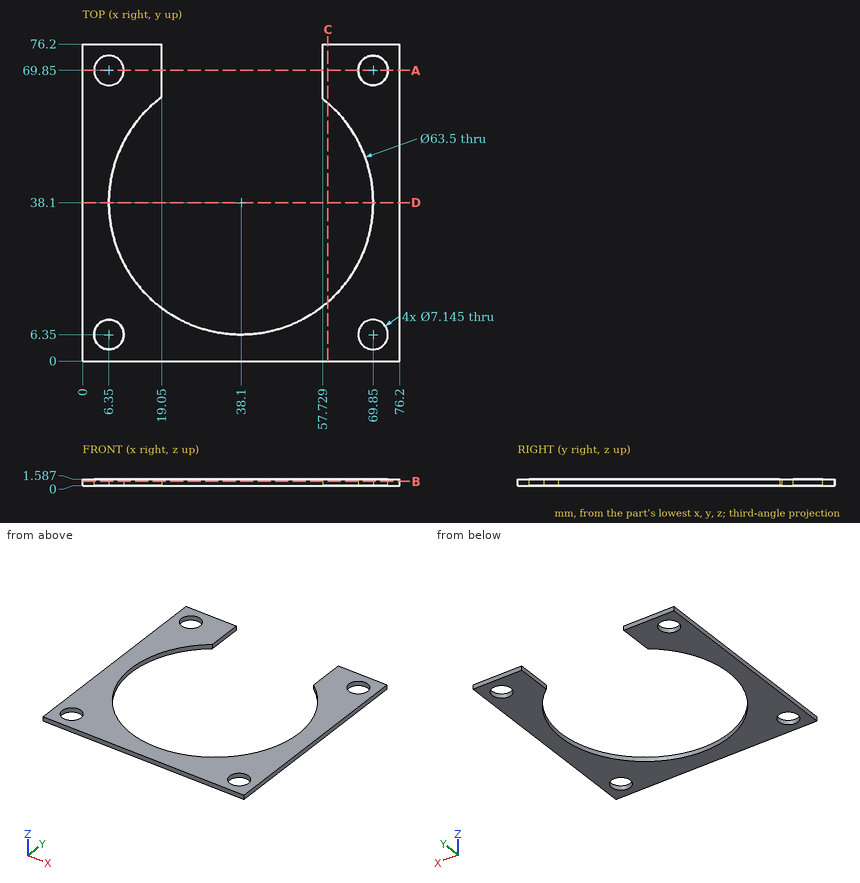
Drawing for the job (mm, zero at the part's lowest x, y, z). Round coordinates to 2 decimals unless told otherwise and drop trailing zeros. Write each loop counter-clockwise with the first axis right and the second up, starting at its lowest first coordinate (ties: lowest second). Pieces come first, ordered by that corner, then holes. Notation, with made-up numbers: M -28.5,-2.75 L -9.5,-2.75 A13 ccw -9.5,11.25 Z; hole C -34,-20.75 d5. An arc over 180 degrees is marked long. Answer as a JSON object with one key per item and string values. Group by question number.
(1) Cut at D-D (y = 38.1). Give the cut face in (x, z).
(2) Cut at B-B (z = 1). Give the number of separate pieces and of enclosed holes in the cut face, and give its area (3 significant figures).
(3) Cut at A-A (y = 69.85). Give the cut face in (x, z).
(4) Drill centre lines: L1, parallel to Y at x = 71, z = 0.95; L2, parallel to X at y = 5, z = 0.65; L3, parallel to X at y = 38.1, z = 0.95. Where is each one in solid material? Low to high.
(5) Cut at C-C (x = 59). Give the cut face in (y, z).
Responses:
{
 "1": {"outline": "M 0,0 L 6.35,0 L 6.35,1.59 L 0,1.59 Z; M 69.85,0 L 76.2,0 L 76.2,1.59 L 69.85,1.59 Z"},
 "2": {"separate pieces": "1", "enclosed holes": "4", "area": "2,150 mm2"},
 "3": {"outline": "M 0,0 L 2.78,0 L 2.78,1.59 L 0,1.59 Z; M 9.92,0 L 19.05,0 L 19.05,1.59 L 9.92,1.59 Z; M 57.73,0 L 66.28,0 L 66.28,1.59 L 57.73,1.59 Z; M 73.42,0 L 76.2,0 L 76.2,1.59 L 73.42,1.59 Z"},
 "4": {"L1": "y = 0 to 2.97, 9.73 to 66.47, 73.23 to 76.2", "L2": "x = 0 to 3.04, 9.66 to 66.54, 73.16 to 76.2", "L3": "x = 0 to 6.35, 69.85 to 76.2"},
 "5": {"outline": "M 0,0 L 14.2,0 L 14.2,1.59 L 0,1.59 Z; M 62,0 L 76.2,0 L 76.2,1.59 L 62,1.59 Z"}
}
